Job drawing, mm, ordinate dimensions from the low corner. One solid piece. A direction names the side the tool comes from. Give positions to 0.01 mm unless a question says otherwise; leave off trailing zeros. Loops run counter-clockwise (first coordinate to the right, second up) from the corner with the lowest first, then second, coordinate; pieces in that order, holes last. Notation, with made-up numbers: M 77,71 L 124,71 A20 ccw 124,87 Z; hole C 87.25,31.25 d5. An arc over 180 degrees is marked long. Answer as CSV lines item,"result".
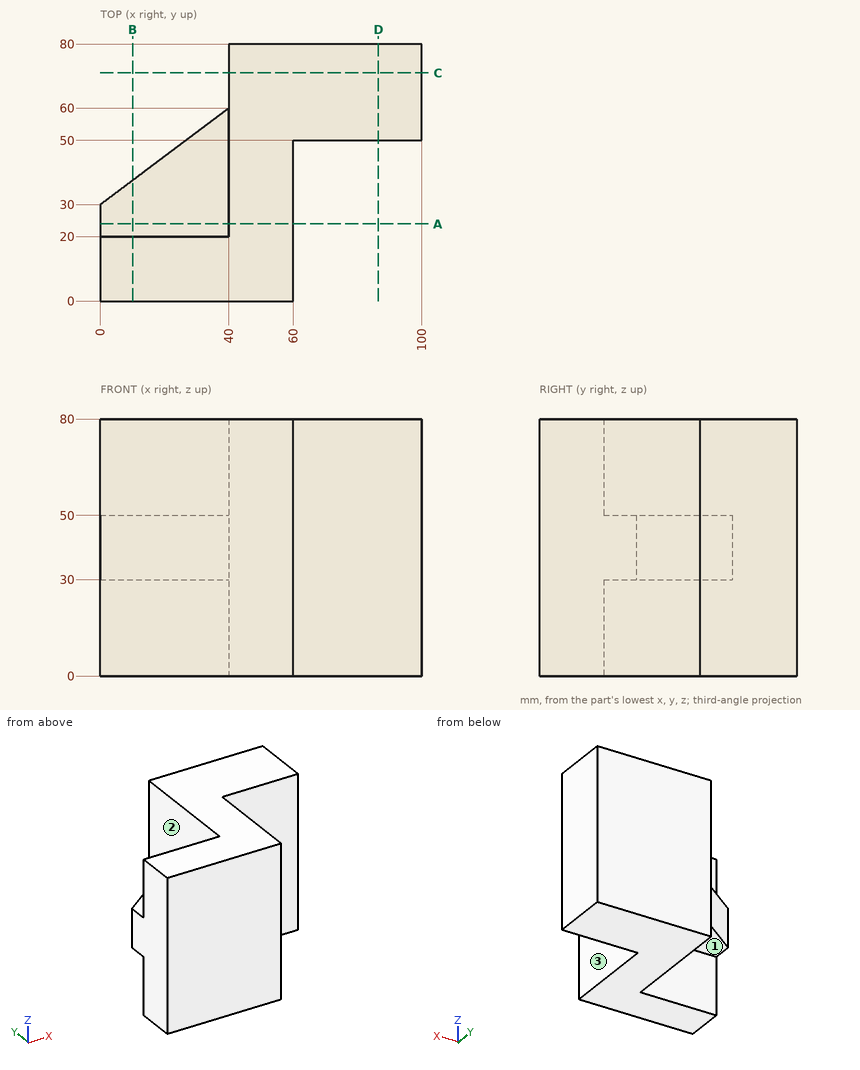
1) Flat gauge pins, fed straight in: pin 1 (8 mm diameter, centred on y = 63.5, z = 35.5, fed in from -X); pin 2 (5 mm diameter, centred on y = 33, z = 63, fed in from +X); pin 3 (9 mm diameter, centred on x = 11, z = 60, fed in from +Y). Where does each tip first touch, or does it go through?
Answer below:
pin 1,"stops at x = 39.33"
pin 2,"stops at x = 60"
pin 3,"stops at y = 20"
2) Which spindle directions (+Z, -Z, +X, -X, +Y, -Y) get a long thin tool onto all of the face, cutting with end or side? Do the marked faces 1, 2 and 3. Say none if no direction does.
Answer below:
face 1,"-Z, -X, +Y"
face 2,"-X, +Y"
face 3,"+Z, -Z, +X, -Y"
3) Band-saw the part on D-D on x = 86.5. Give the cut face in (y, z).
Answer below:
outline,"M 50,0 L 80,0 L 80,80 L 50,80 Z"
4) Band-saw the part on C-C on y = 71. Give the cut face in (x, z), and give its area (3 significant figures).
Answer below:
outline,"M 40,0 L 100,0 L 100,80 L 40,80 Z"
area,"4,800 mm^2"
5) Drill centre lines: line 1 (X direction, y = 30, z = 9); line 2 (X direction, y = 74.5, z = 67.5); line 3 (Y direction, x = 17, z = 29). Where is each one in solid material? Low to high. Write a range as from..to.
Answer below:
line 1,"x = 40..60"
line 2,"x = 40..100"
line 3,"y = 0..20"
6) Band-saw the part on A-A on y = 24. Give the cut face in (x, z), and give its area (3 significant figures).
Answer below:
outline,"M 0,30 L 40,30 L 40,0 L 60,0 L 60,80 L 40,80 L 40,50 L 0,50 Z"
area,"2,400 mm^2"
7) Band-saw the part on B-B on x = 10. Give the cut face in (y, z).
Answer below:
outline,"M 0,0 L 20,0 L 20,30 L 37.5,30 L 37.5,50 L 20,50 L 20,80 L 0,80 Z"
